```python
from build123d import *

# Parameters (mm, degrees)
F_10_0_10_DIAMETER_HOLE1_D     = 10
F_10_0_10_DIAMETER_HOLE1_DEPTH = 2
F_10_0_10_DIAMETER_HOLE1_TIP   = 3.004303095


with BuildPart() as part:
    # Sketch1 → Revolve1 (revolve)
    with BuildSketch(Plane.XY, mode=Mode.PRIVATE) as revolve1_sk:
        with BuildLine():
            Line((17, 0), (17, 6.845299462))
            Line((17, 6.845299462), (15, 8))
            Line((15, 8), (13, 8))
            Line((13, 8), (13, 7))
            Line((13, 7), (11, 7))
            Line((11, 7), (11, 8))
            Line((11, 8), (4, 8))
            ThreePointArc((4, 8), (1.05572809, 4.472135955), (0, 0))
            Line((0, 0), (17, 0))
        make_face()
    revolve(revolve1_sk.sketch.rotate(Axis((0, 0, 0), (1, 0, 0)), 90), axis=Axis((0, 0, 0), (1, 0, 0)))

    # Ø10.0 (10) Diameter Hole1
    with Locations(Plane(origin=(17, 0, 0), x_dir=(0, 0, -1), z_dir=(1, 0, 0))):
        with Locations((0, 0)):
            Hole(F_10_0_10_DIAMETER_HOLE1_D / 2, depth=F_10_0_10_DIAMETER_HOLE1_DEPTH)
            with Locations((0, 0, -(F_10_0_10_DIAMETER_HOLE1_DEPTH + F_10_0_10_DIAMETER_HOLE1_TIP / 2))):  # 118° drill point
                Cone(0, F_10_0_10_DIAMETER_HOLE1_D / 2, F_10_0_10_DIAMETER_HOLE1_TIP, mode=Mode.SUBTRACT)


solid = part.part
```
The model under review builds one solid part; all positions refer to its coordinate system, in mm. A direction names the side the tool comes from. Round coordinates to 2 decimals unless told otherwise and drop trailing zeros. Loops run counter-clockwise (first coordinate to the right, second up) from the corner with the lowest first, then second, coordinate; pieces in that order, holes last. Notation, with made-up numbers: (78.25, -39.75) -> (112.25, -39.75) arc R13 ccw to (112.25, -32.75) -> close; hole circle Ø5 at (-11.75, 24). An arc over 180 degrees is marked (long way). Answer as a JSON object with one key per item and string values. Group by question number.
1) We need section B-B on x = 13.5. Write out the cut boundary in (y, z).
2) For line 1 (Y direction, x = 16.35, z = 0); line 2 (Y direction, x = 14.75, z = 0.75); line 3 (X direction, y = 6.5, z = -3.5), list the stretches that pass through material, from the lowest coordinate up. Write a range as [from, to].
3) We need section A-A on x = 4.5. Write out the cut boundary in (y, z).
4) Mouldability with a two-part tool opening along Y and no side actions: class faces 4 (the face through (17, 2, 5)), 5 (the face through (11.99, 6.21, 3.23)), 6 (the face through (12.52, -0.85, 0.19)) as released by +Y, released by -Y, zero draft, split by the parting line, or undercut.
5) For faces 1 (the face through (15.99, -4.88, -1.08)), 2 (the face through (11, 6, -4)), 3 (the face through (13.99, 7.81, -1.73)), list the 3-axis set-ups (+Z, -Z, +X, -X, +Y, -Y) from which the entire face can be reached by the end or side of a thin tool; tool diameter is ignored.
6) For pin 1 Ø1.5 at (y, z) = (3.5, 2.5) entering from +X, flat-tipped, find the tip position at first contact; note if it passes through.
Result set:
{
 "1": {"outline": "circle Ø16 at (0, 0); hole circle Ø5.01 at (0, 0)"},
 "2": {"line 1": "[-7.22, -5], [5, 7.22]", "line 2": "[-7.96, -4.52], [4.52, 7.96]", "line 3": "[3.25, 11], [13, 16.07]"},
 "3": {"outline": "circle Ø16 at (0, 0)"},
 "4": {"face 4": "zero draft", "face 5": "split by the parting line", "face 6": "undercut"},
 "5": {"face 1": "+X", "face 2": "none", "face 3": "+X, -X"},
 "6": {"pin 1": "x = 17"}
}
